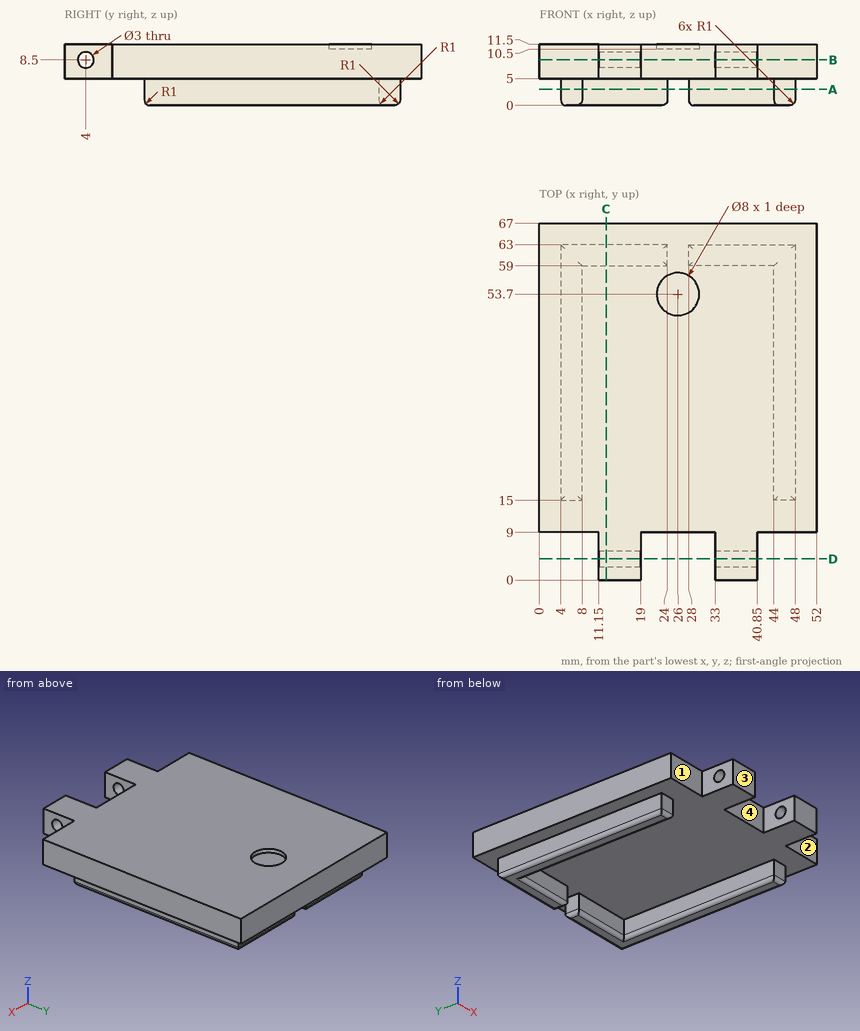
Drawing for the job (mm, zero at the part's lowest x, y, z). A direction names the side the tool comes from. Coordinates: 2 decimals unless noted, no trailing zeros. Write each loop counter-clockwise with the first axis right and the second up, starting at its lowest first coordinate (ties: lowest second). Pieces come first, ordered by that corner, then holes. Notation, with made-up numbers: (22, 34) - (29, 34) arc R5 ccw to (29, 38) - close; hole circle Ø2 at (-13, 5.5). An arc over 180 degrees is marked (long way). Write each question's results on one line, items separated by ' | '. Start each with the question number.
1) Cut at B-B (z = 8.5). Write the cut outline in (x, y).
2) Cut at D-D (y = 4). Write the cut outline in (x, z).
3) 3-axis set-ups, long thin cutter, end or side, ignore diameter. For the marked faces 1, 2, 3 and 4: which of +Z, -Z, +X, -X, +Y, -Y reach the whole face in a straight line?
4) Cut at C-C (x = 12.5). Write the cut outline in (y, z).
5) Probe line 1 along X through (y, z) = (4, 6.5); line 2 along Y through (x, z) = (26, 11.2); line 3 along X through (y, z) = (42.5, 4.75). List the from-to ranges inside material, lowest first. Write a range as from..to.
6) Cut at A-A (z = 3). Write the cut outline in (x, y).
7) Flat gauge pins, fed straight in: P1, Ø1.2, axis at y = 61.5, z = 3.5, coming from the -X side; P2, Ø5, axis at x = 28.5, z = 7.5, coming from the -Y side; P3, Ø8, axis at x = 19, y = 15, coming from the -Z side. Where does each tip first touch, or does it go through?
Returned:
1) outline: (0, 9) - (11.15, 9) - (11.15, 5.5) - (19, 5.5) - (19, 9) - (33, 9) - (33, 5.5) - (40.85, 5.5) - (40.85, 9) - (52, 9) - (52, 67) - (0, 67) - close; (11.15, 0) - (19, 0) - (19, 2.5) - (11.15, 2.5) - close; (33, 0) - (40.85, 0) - (40.85, 2.5) - (33, 2.5) - close
2) outline: (11.15, 5) - (19, 5) - (19, 7) - (11.15, 7) - close; (11.15, 10) - (19, 10) - (19, 11.5) - (11.15, 11.5) - close; (33, 5) - (40.85, 5) - (40.85, 7) - (33, 7) - close; (33, 10) - (40.85, 10) - (40.85, 11.5) - (33, 11.5) - close
3) face 1: +Z, -Z, -X, -Y | face 2: +Z, -Z, +X, -Y | face 3: +Z, -Z, +X, -X, -Y | face 4: +Z, -Z, -Y
4) outline: (0, 5) - (59, 5) - (59, 1) arc R1 ccw to (60, 0) - (62, 0) arc R1 ccw to (63, 1) - (63, 5) - (67, 5) - (67, 11.5) - (0, 11.5) - close; hole circle Ø3 at (4, 8.5)
5) line 1: 11.15..19, 33..40.85 | line 2: 9..49.7, 57.7..67 | line 3: 4..8, 44..48
6) outline: (4, 15) - (8, 15) - (8, 59) - (24, 59) - (24, 63) - (4, 63) - close; (28, 59) - (44, 59) - (44, 15) - (48, 15) - (48, 63) - (28, 63) - close
7) P1: x = 4 | P2: y = 9 | P3: z = 5
